The listing builds one solid part. Answer for the finished solid, in the listing's coordinates (mm). Face numbers are marked on the shaded views. A direction names the side the tool comes from. Round coordinates to 2 decimals unless told otherwise and drop trailing zeros. Write each loop counter-clockwise with the first axis right and the second up, starting at its lowest first coordinate (ties: lowest second). Pieces come first, ordered by that corner, then holes.
Item 1: This flat-tipped pin is pushed along its axis until it touches: pin 1 (1.5 mm diameter, centred on x = -7.5, y = -22.5, fed in from +Z). Where does it stop, or does it pass through?
Item 2: Find section D-D on x = 8.5. Give the vertices of the cut face in (y, z).
Item 3: Find section A-A on z = -9.5. Give the vertices of the cut face in (x, y), then the cut area to 3 significant figures.
Item 4: Find the intervals of material crossed by probe 1 along Z at (x, y) = (29, -11.75); probe 2 along Z at (x, y) = (-25.5, -16.75); probe 3 along Z at (x, y) = (17, -3), in increasing order.
Item 5: Find section C-C on z = -38. Give the vertices of the cut face in (x, y).
Item 6: For a pull along Z with two mould halves and no side action, classify the marked faces 3 and 4 as +Z half, -Z half, draft (parallel to the pull), parting line (faces both ways), or undercut.
Item 7: Find section B-B on x = -25. Give the vertices of the cut face in (y, z).
Item 8: A tool of negligible diameter and unlimited length cuts with its end or side. For the marked faces 1 and 2, from which of +Z, -Z, +X, -X, +Y, -Y can it reach the whole face along a straight path? Write none if from no direction.
```python
from build123d import *

# Parameters (mm, degrees)
F0_R     = 5
F1_DEPTH = 25


with BuildPart() as f1:
    # F0 (on Front) → F1 (new body)
    with BuildSketch(Plane.XZ):
        with BuildLine():
            ThreePointArc((0, 75), (-24.748737, 64.748737), (-35, 40))
            Line((-35, 40), (-35, 0))
            Line((-35, 0), (-35, -40))
            ThreePointArc((-35, -40), (-24.748737, -64.748737), (0, -75))
            ThreePointArc((0, -75), (24.748737, -64.748737), (35, -40))
            Line((35, -40), (35, 0))
            Line((35, 0), (35, 40))
            ThreePointArc((35, 40), (24.748737, 64.748737), (0, 75))
        make_face()
        with Locations((-17.67767, -57.67767)):
            Circle(F0_R, mode=Mode.SUBTRACT)
        with Locations((-25, -40)):
            Circle(F0_R, mode=Mode.SUBTRACT)
        with Locations((-25, -20)):
            Circle(F0_R, mode=Mode.SUBTRACT)
        with Locations((0, -65)):
            Circle(F0_R, mode=Mode.SUBTRACT)
        with Locations((17.67767, -57.67767)):
            Circle(F0_R, mode=Mode.SUBTRACT)
        with Locations((25, -40)):
            Circle(F0_R, mode=Mode.SUBTRACT)
        with Locations((25, -20)):
            Circle(F0_R, mode=Mode.SUBTRACT)
        with Locations((-25, 0)):
            Circle(F0_R, mode=Mode.SUBTRACT)
        with Locations((-25, 20)):
            Circle(F0_R, mode=Mode.SUBTRACT)
        with Locations((-25, 40)):
            Circle(F0_R, mode=Mode.SUBTRACT)
        with Locations((-17.67767, 57.67767)):
            Circle(F0_R, mode=Mode.SUBTRACT)
        with BuildLine():
            ThreePointArc((-15, 40), (-10.606602, 50.606602), (0, 55))
            ThreePointArc((0, 55), (10.606602, 50.606602), (15, 40))
            Line((15, 40), (15, 0))
            Line((15, 0), (15, -40))
            ThreePointArc((15, -40), (10.606602, -50.606602), (0, -55))
            ThreePointArc((0, -55), (-10.606602, -50.606602), (-15, -40))
            Line((-15, -40), (-15, 0))
            Line((-15, 0), (-15, 40))
        make_face(mode=Mode.SUBTRACT)
        with Locations((25, 0)):
            Circle(F0_R, mode=Mode.SUBTRACT)
        with Locations((25, 20)):
            Circle(F0_R, mode=Mode.SUBTRACT)
        with Locations((0, 65)):
            Circle(F0_R, mode=Mode.SUBTRACT)
        with Locations((25, 40)):
            Circle(F0_R, mode=Mode.SUBTRACT)
        with Locations((17.67767, 57.67767)):
            Circle(F0_R, mode=Mode.SUBTRACT)
    extrude(amount=F1_DEPTH)


solid = f1.part
```
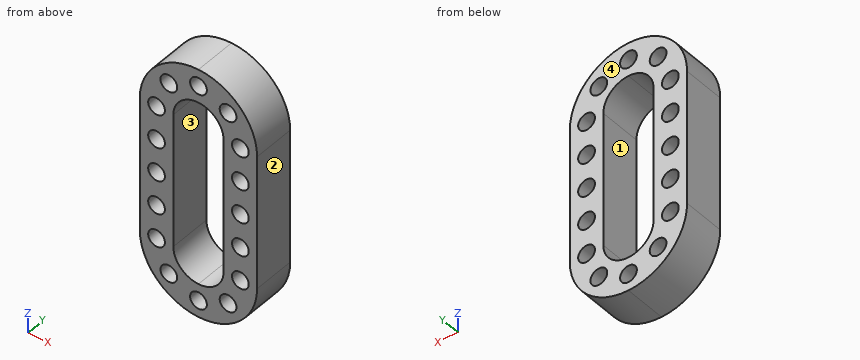
Check values:
1. pin 1: stops at z = 74.34
2. outline: (-25, -73.95) - (0, -73.95) - (0, -52.36) - (-25, -52.36) - close; (-25, 52.36) - (0, 52.36) - (0, 73.95) - (-25, 73.95) - close
3. outline: (-35, -25) - (-15, -25) - (-15, 0) - (-35, 0) - close; (15, -25) - (35, -25) - (35, 0) - (15, 0) - close
3. area: 1,000 mm2
4. probe 1: z = -59.6 to -43, -37 to -23, -17 to -3, 3 to 17, 23 to 37, 43 to 59.6
4. probe 2: z = -63.97 to -44.97, -35.03 to -24.97, -15.03 to -4.97, 4.97 to 15.03, 24.97 to 35.03, 44.97 to 63.97
4. probe 3: z = -70.59 to -62.63, -52.72 to 52.72, 62.63 to 70.59
5. outline: (-35, -25) - (-29.58, -25) - (-29.58, 0) - (-35, 0) - close; (-20.42, -25) - (-15, -25) - (-15, 0) - (-20.42, 0) - close; (15, -25) - (20.42, -25) - (20.42, 0) - (15, 0) - close; (29.58, -25) - (35, -25) - (35, 0) - (29.58, 0) - close
6. face 3: undercut
6. face 4: draft
7. outline: (-25, -64.49) - (0, -64.49) - (0, -45) - (-25, -45) - close; (-25, -35) - (0, -35) - (0, -25) - (-25, -25) - close; (-25, -15) - (0, -15) - (0, -5) - (-25, -5) - close; (-25, 5) - (0, 5) - (0, 15) - (-25, 15) - close; (-25, 25) - (0, 25) - (0, 35) - (-25, 35) - close; (-25, 45) - (0, 45) - (0, 64.49) - (-25, 64.49) - close
8. face 1: +Y, -Y
8. face 2: +Z, -Z, +X, +Y, -Y
